Part model, mm, in its own coordinate system. Give positions to 0.01 mm unless a question says otherwise; leave off trailing zeros. Order: outer loops, then holes, each group sorted by start corner. A loop starts at its lowest first (then second) coordinate and runs counter-clockwise, first axis right, second up. Notation, with made-up numbers: (27, 85) - (86, 85) arc R19 ccw to (86, 114) - close; hole circle Ø7 at (78, 17). An arc over 180 degrees is marked (long way). Use a Markdown table: item, result. Add a question column.
from build123d import *

# Parameters (mm, degrees)
SKETCH_1_R          = 82.5
EXTRUDE_1_DEPTH     = 2
SKETCH_2_R          = 3.8
SKETCH_2_R_2        = 5
CUT_EXTRUDE_1_DEPTH = 117.689759619


with BuildPart() as part:
    # 草图1 → 凸台-拉伸1 (new body)
    with BuildSketch(Plane.XY):
        Circle(SKETCH_1_R)
    extrude(amount=EXTRUDE_1_DEPTH)

    # 草图2 → 切除-拉伸1 (cut, through all)
    with BuildSketch(Plane.XY.offset(2)):
        with Locations((30, 30)):
            Circle(SKETCH_2_R)
        with Locations((-30, 30)):
            Circle(SKETCH_2_R)
        with Locations((-30, -30)):
            Circle(SKETCH_2_R)
        with Locations((30, -30)):
            Circle(SKETCH_2_R)
        Circle(SKETCH_2_R_2)
    extrude(amount=-CUT_EXTRUDE_1_DEPTH, mode=Mode.SUBTRACT)


solid = part.part
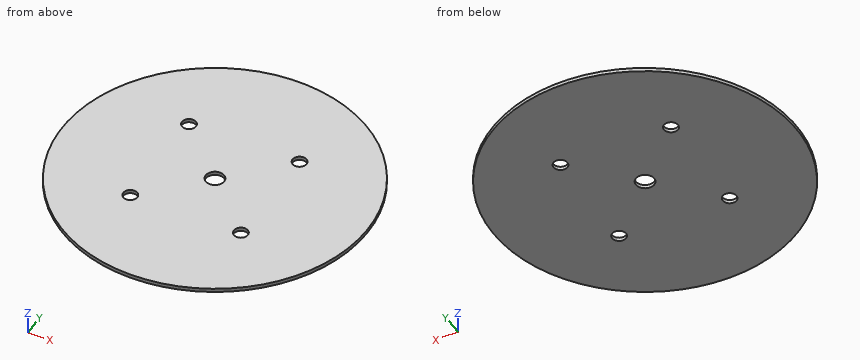
1. Pin check, flat tips, straight feed: P1, Ø1, axis at x = -16, z = 1, coming from the -Y side; P2, Ø1, axis at x = 47.5, z = 1.5, coming from the +Y side; P3, Ø6, axis at x = -30, y = 30, coming from the -Z side. Stop position of each tip, or through.
2. Cut at A-A (x = 0). Write the cut outline in (y, z), plus the area to 3 significant figures.
3. Drill centre lines: probe 1 along Y at (x, z) = (0, 0.75); probe 2 along Y at (x, z) = (30, 1.55); probe 3 along Y at (x, z) = (-26.5, 1.7). Where is each one in solid material? Low to high. Write a range as [from, to].
4. Cut at C-C (y = -30). Write the cut outline in (x, z).
Responses:
| question | item | result |
|---|---|---|
| 1 | P1 | stops at y = -81.03 |
| 1 | P2 | stops at y = 67.8 |
| 1 | P3 | passes through |
| 2 | outline | (-82.5, 0) - (-5, 0) - (-5, 2) - (-82.5, 2) - close; (5, 0) - (82.5, 0) - (82.5, 2) - (5, 2) - close |
| 2 | area | 310 mm² |
| 3 | probe 1 | y = [-82.5, -5], [5, 82.5] |
| 3 | probe 2 | y = [-76.85, -33.8], [-26.2, 26.2], [33.8, 76.85] |
| 3 | probe 3 | y = [-78.13, -31.48], [-28.52, 28.52], [31.48, 78.13] |
| 4 | outline | (-76.85, 0) - (-33.8, 0) - (-33.8, 2) - (-76.85, 2) - close; (-26.2, 0) - (26.2, 0) - (26.2, 2) - (-26.2, 2) - close; (33.8, 0) - (76.85, 0) - (76.85, 2) - (33.8, 2) - close |
